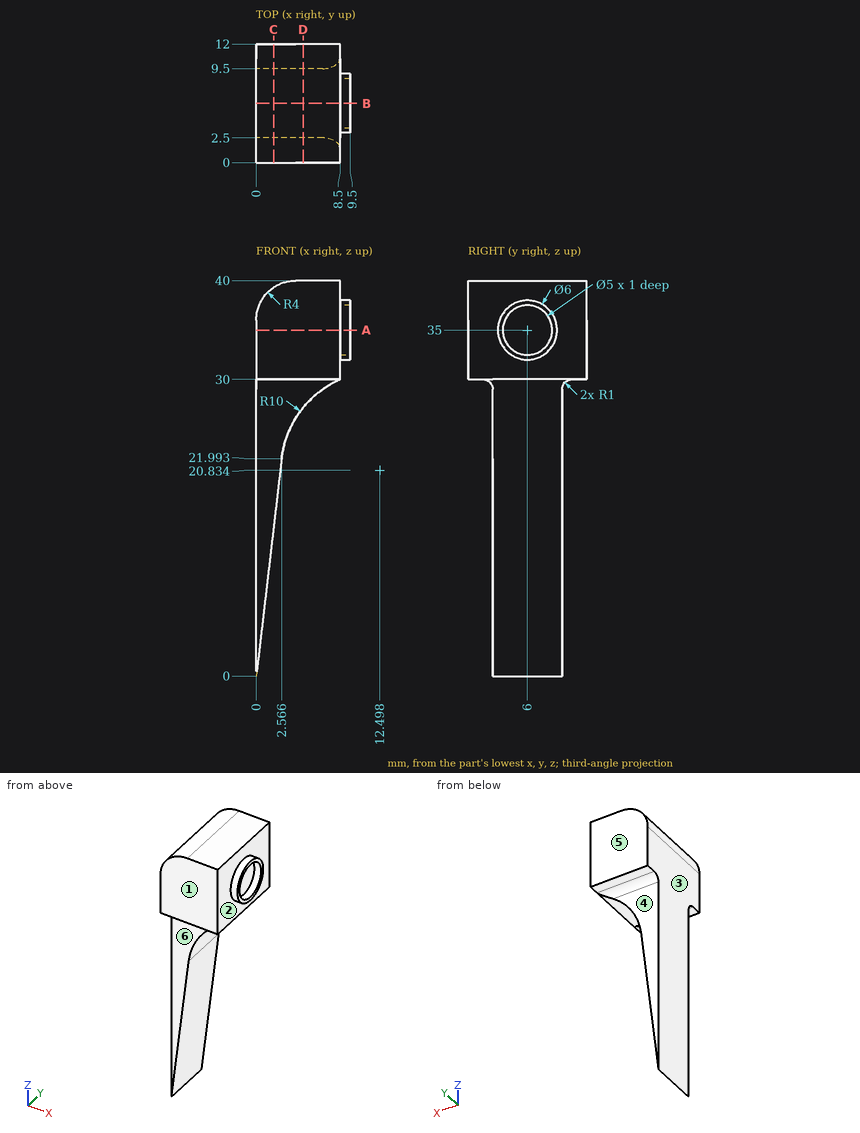
Job drawing, mm, ordinate dimensions from the low corner. One solid piece. A direction names the side the tool comes from. Coordinates: 2 decimals unless noted, no trailing zeros. Loops run counter-clockwise (first coordinate to the right, second up) from the corner with the lowest first, then second, coordinate; pieces in that order, holes last. Notation, with made-up numbers: (83.5, -13) - (108.5, -13) arc R36 cw to (108.5, 21) - close; hole circle Ø1 at (33, 38.25). An arc over 180 degrees is marked (long way). Write item = value, one per line. Start each with the question number.
Q1. Flat gauge pins, fed straight in: pin 1 Ø2.5 at (y, z) = (5, 34.5) entering from +X; pin 2 Ø1.2 at (x, y) = (4.5, 11) entering from -Z (1 decimal). Where does each tip first touch, or does it go through?
Q2. Pull direction X, two halves, no side cores. Call the marked faces 1, 2 and 3: pulls with the +X half, pulls with the -X half, needs draft (parallel to the pull), parting line crosses it, or undercut.
Q3. Cut at D-D, the plane x = 4.75. List the corners of the cut face in (y, z) (1 decimal).
Q4. Drill centre lines: L1, parallel to Y at x = 8.85, z = 35; L2, parallel to Y at x = 1.75, z = 24.5; L3, parallel to X at y = 5.5, z = 30.5. Where is each one in solid material? Low to high.
Q5. Cut at A-A, the plane z = 35. List the corners of the cut face in (x, y), then the cut area to 3 significant figures.
Q6. Cut at B-B, the plane y = 6. List the corners of the cut face in (x, z) (1 decimal), then the cut area to 3 significant figures.
Q7. Which spindle directions (+Z, -Z, +X, -X, +Y, -Y) get a long thin tool onto all of the face, cutting with end or side? Do the marked faces 4, 5 and 6. Say none if no direction does.
Q8. Cut at C-C, the plane x = 1.75. List the corners of the cut face in (y, z).
Computed:
q1.pin_1 = 8.5
q1.pin_2 = 30
q2.face_1 = needs draft
q2.face_2 = pulls with the +X half
q2.face_3 = pulls with the -X half
q3.outline = (0, 30) - (1.5, 30) arc R1 cw to (2.5, 29) - (2.5, 27.2) - (9.5, 27.2) - (9.5, 29) arc R1 cw to (10.5, 30) - (12, 30) - (12, 40) - (0, 40) - close
q4.L1 = 3 to 3.5, 8.5 to 9
q4.L2 = 2.5 to 9.5
q4.L3 = 0 to 8.5
q5.outline = (0, 0) - (8.5, 0) - (8.5, 3) - (9.5, 3) - (9.5, 3.5) - (8.5, 3.5) - (8.5, 8.5) - (9.5, 8.5) - (9.5, 9) - (8.5, 9) - (8.5, 12) - (0, 12) - close
q5.area = 103 mm²
q6.outline = (0, 0) - (2.6, 22) arc R10 cw to (8.5, 30) - (8.5, 32) - (9.5, 32) - (9.5, 32.5) - (8.5, 32.5) - (8.5, 37.5) - (9.5, 37.5) - (9.5, 38) - (8.5, 38) - (8.5, 40) - (4, 40) arc R4 ccw to (0, 36) - close
q6.area = 146 mm²
q7.face_4 = -Z, +X, -X, +Y
q7.face_5 = +Z, -Z, +X, -X, +Y
q7.face_6 = -Z, +X, -X, -Y
q8.outline = (0, 30) - (1.5, 30) arc R1 cw to (2.5, 29) - (2.5, 15) - (9.5, 15) - (9.5, 29) arc R1 cw to (10.5, 30) - (12, 30) - (12, 39.31) - (0, 39.31) - close
